```python
from build123d import *

# Parameters (mm, degrees)
F0_W     = 50
F0_H     = 6
F0_R     = 1.75
F1_DEPTH = 2
F2_R     = 0.4
F3_DEPTH = 2.001


with BuildPart() as f1:
    # F0 (on Top) → F1 (new body)
    with BuildSketch(Plane.XY):
        with Locations((25, 3)):
            Rectangle(F0_W, F0_H)
        with Locations((3.25, 3)):
            Circle(F0_R, mode=Mode.SUBTRACT)
        with Locations((46.75, 3)):
            Circle(F0_R, mode=Mode.SUBTRACT)
    extrude(amount=F1_DEPTH)

    # F2 (on face) → F3 (cut, through all)
    with BuildSketch(Plane.XY.offset(2)):
        with Locations((11.25, 5)):
            Circle(F2_R)
        with Locations((15.25, 5)):
            Circle(F2_R)
        with Locations((19.25, 5)):
            Circle(F2_R)
        with Locations((23.25, 5)):
            Circle(F2_R)
        with Locations((27.25, 5)):
            Circle(F2_R)
        with Locations((31.25, 5)):
            Circle(F2_R)
        with Locations((35.25, 5)):
            Circle(F2_R)
        with Locations((38.75, 5)):
            Circle(F2_R)
    extrude(amount=-F3_DEPTH, mode=Mode.SUBTRACT)


solid = f1.part
```
Verification items for the finished model (mm, model axes). Coordinates: 2 decimals unless noted, no trailing zeros. Order: outer loops, then holes, each group sorted by start corner. A loop starts at its lowest first (then second) coordinate and runs counter-clockwise, first axis right, second up. Notation, with made-up numbers: (-24, -32.5) - (2, -32.5) arc R26 cw to (2, -5.5) - close; hole circle Ø3 at (68, -7.75). An arc over 180 degrees is marked (long way). Return JSON: item names as keys, results as strings.
(1) Section check C-C, the plane y = 3. Record the cut outline in (x, z), and give its area (3 significant figures).
Filled sheet:
{"outline": "(0, 0) - (1.5, 0) - (1.5, 2) - (0, 2) - close; (5, 0) - (45, 0) - (45, 2) - (5, 2) - close; (48.5, 0) - (50, 0) - (50, 2) - (48.5, 2) - close", "area": "86.0 mm^2"}
(2) Thickness scan on line 1 along X through (y, z) = (4.4, 1.55); line 2 along Y through (x, z) = (35.25, 0.75); line 3 along X through (y, z) = (1.4, 1.35). Record the ranges inside material, lowest first.
Filled sheet:
{"line 1": "x = 0 to 2.2, 4.3 to 45.7, 47.8 to 50", "line 2": "y = 0 to 4.6, 5.4 to 6", "line 3": "x = 0 to 2.54, 3.96 to 46.04, 47.46 to 50"}
(3) Section check A-A, the plane x = 3.25. Record the cut outline in (y, z).
Filled sheet:
{"outline": "(0, 0) - (1.25, 0) - (1.25, 2) - (0, 2) - close; (4.75, 0) - (6, 0) - (6, 2) - (4.75, 2) - close"}
(4) Section check B-B, the plane z = 1.5. Give the number of separate pieces and of enclosed holes in the cut face, and give its area (3 significant figures).
Filled sheet:
{"separate pieces": "1", "enclosed holes": "10", "area": "277 mm^2"}
(5) Mould release check, pull along X, two halves, no side actions. Record for faces 1 (the cylindrical face through (15.63, 5.12, 1.01)), 2 (the flat face through (25, 6, 1)), 3 (the flat face through (50, 3, 1)): pulls with the +X half, pulls with the -X half, needs draft (parallel to the pull), parting line crosses it, or undercut.
Filled sheet:
{"face 1": "undercut", "face 2": "needs draft", "face 3": "pulls with the +X half"}
